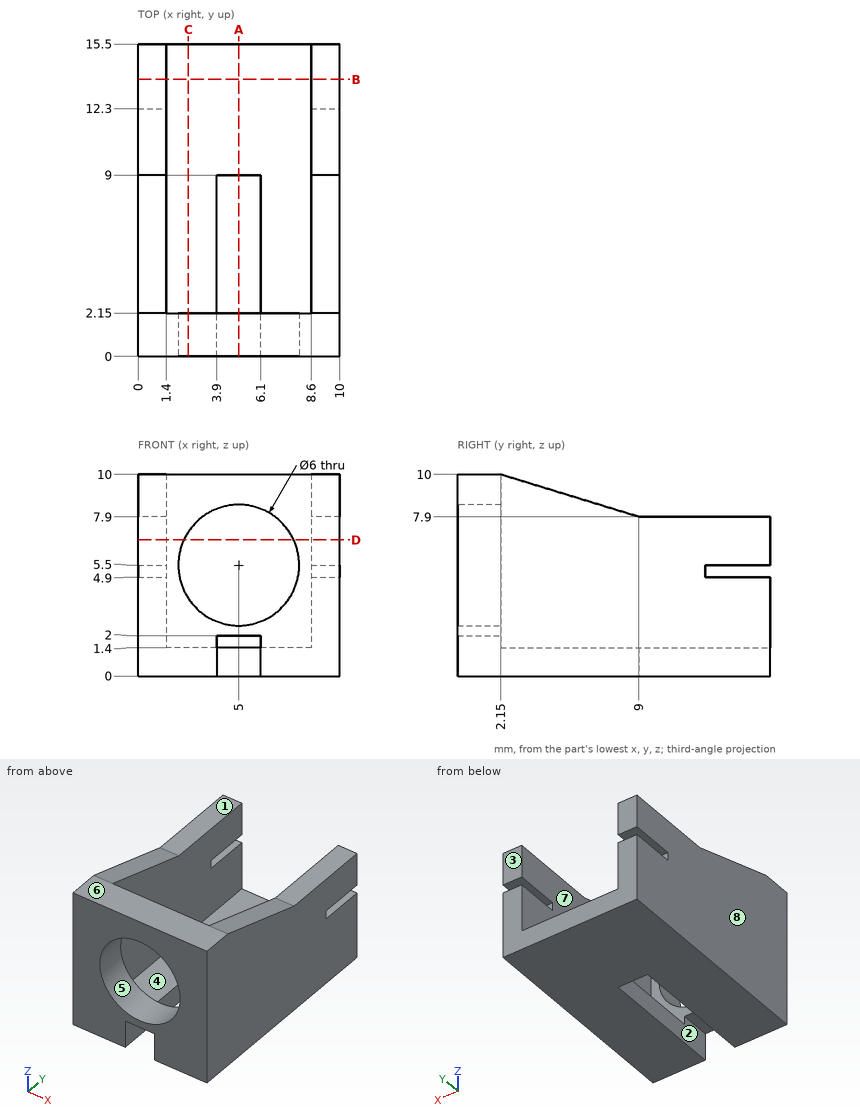
Check sheet for the drawn part. Datum: minimum x, y, z corner. Units: mm. A direction names the side the tool comes from. Coordinates: 2 decimals unless noted, no trailing zeros. Loops run counter-clockwise (first coordinate to the right, second up) from the corner with the lowest first, then second, coordinate; pieces in that order, holes last. Notation, with made-up numbers: (-26, 84) -> (9, 84) arc R26 ccw to (9, 111) -> close; hole circle Ø10 at (80.5, 83). An arc over 180 degrees is marked (long way). Answer in a Markdown table with one row per item.
1) Scan lines: line 1 along X through (y, z) = (0.9, 5.5); line 2 along X through (y, z) = (4.5, 4.25); line 3 along Y through (x, z) = (3.25, 2.5). Record each from-to range of solid material in increasing order. Write a range as from..to.
The answers:
| item | result |
|---|---|
| line 1 | x = 0..2, 8..10 |
| line 2 | x = 0..1.4, 8.6..10 |
| line 3 | y = 0..2.15 |
2) Section check C-C (x = 2.5). Record the cut outline in (y, z), and give its area (3 significant figures).
The answers:
| item | result |
|---|---|
| outline | (0, 0) -> (15.5, 0) -> (15.5, 1.4) -> (2.15, 1.4) -> (2.15, 3.84) -> (0, 3.84) -> close; (0, 7.16) -> (2.15, 7.16) -> (2.15, 10) -> (0, 10) -> close |
| area | 33.1 mm2 |
3) Section check A-A (x = 5). Record the cut outline in (y, z), and give its area (3 significant figures).
The answers:
| item | result |
|---|---|
| outline | (0, 2) -> (2.15, 2) -> (2.15, 2.5) -> (0, 2.5) -> close; (0, 8.5) -> (2.15, 8.5) -> (2.15, 10) -> (0, 10) -> close; (9, 0) -> (15.5, 0) -> (15.5, 1.4) -> (9, 1.4) -> close |
| area | 13.4 mm2 |
4) Section check D-D (z = 6.75). Record the cut outline in (x, y).
The answers:
| item | result |
|---|---|
| outline | (0, 0) -> (2.27, 0) -> (2.27, 2.15) -> (1.4, 2.15) -> (1.4, 15.5) -> (0, 15.5) -> close; (7.73, 0) -> (10, 0) -> (10, 15.5) -> (8.6, 15.5) -> (8.6, 2.15) -> (7.73, 2.15) -> close |
5) Section check B-B (y = 13.75). Record the cut outline in (x, z), and give its area (3 significant figures).
The answers:
| item | result |
|---|---|
| outline | (0, 0) -> (10, 0) -> (10, 4.9) -> (8.6, 4.9) -> (8.6, 1.4) -> (1.4, 1.4) -> (1.4, 4.9) -> (0, 4.9) -> close; (0, 5.5) -> (1.4, 5.5) -> (1.4, 7.9) -> (0, 7.9) -> close; (8.6, 5.5) -> (10, 5.5) -> (10, 7.9) -> (8.6, 7.9) -> close |
| area | 30.5 mm2 |
6) Draft check along X on the marked faces 6, 7 and 8. Enter one of: released by +X, released by -X, zero draft, split by the parting line, or undercut.
The answers:
| item | result |
|---|---|
| face 6 | zero draft |
| face 7 | undercut |
| face 8 | released by -X |
7) Depth check by flat-ended pin: P1, Ø1.1, axis at x = 1, y = 14, coming from the +Z side; P2, Ø1.1, axis at x = 5, z = 0.5, coming from the -Y side; P3, Ø2, axis at x = 6.5, z = 5, coming from the -Y side. Enter the tip coordinate at first touch or a pass-through.
The answers:
| item | result |
|---|---|
| P1 | stops at z = 7.9 |
| P2 | stops at y = 9 |
| P3 | passes through |
8) Access from +Z, -Z, +X, -X, +Y, -Y to the whole of each face (thin tool, end or side, straight path). Record for the marked faces 1, 2, 3, 4 and 5.
The answers:
| item | result |
|---|---|
| face 1 | +Z, +X, -X, +Y |
| face 2 | -Z, -Y |
| face 3 | +Z, -Z, +X, -X, +Y |
| face 4 | +Z, +Y |
| face 5 | +Y, -Y |
